Design review of the part built by this model. Coordinates are the model's own, in mm. A direction names the side the tool comes from. Coordinates: 2 decimals unless noted, no trailing zeros. Loops run counter-clockwise (first coordinate to the right, second up) from the corner with the lowest first, then second, coordinate; pieces in that order, holes last. Notation, with made-up numbers: (60.5, 6.5) - (101.5, 6.5) arc R31 cw to (101.5, 43.5) - close; hole circle Ø1 at (30.25, -35). An arc over 180 degrees is marked (long way). Return JSON: item names as keys, results as strings. Group by question number.
from build123d import *

# Parameters (mm, degrees)
BOSS_EXTRUDE1_DEPTH  = 15
SKETCH2_R            = 12.5
BOSS_EXTRUDE2_DEPTH  = 35
FILLET1_R            = 2
SKETCH3_R            = 10
BOSS_EXTRUDE3_DEPTH  = 15
FILLET1_OF_MIRROR1_R = 2


with BuildPart() as part:
    # Sketch1 → Boss-Extrude1 (new body)
    with BuildSketch(Plane.XY):
        with BuildLine():
            Line((-12.5, 50), (-12.5, 21.650635095))
            ThreePointArc((-12.5, 21.650635095), (0, -25), (12.5, 21.650635095))
            Line((12.5, 21.650635095), (12.5, 50))
            ThreePointArc((12.5, 50), (0, 62.5), (-12.5, 50))
        make_face()
    boss_extrude1 = extrude(amount=BOSS_EXTRUDE1_DEPTH)

    # Sketch2 → Boss-Extrude2 (add)
    with BuildSketch(Plane.XY.offset(15)):
        Circle(SKETCH2_R)
    boss_extrude2 = extrude(amount=BOSS_EXTRUDE2_DEPTH)

    # Fillet1
    fillet1_edges = [part.edges().sort_by_distance(p)[0] for p in [
        (-12.5, 0, 15),
    ]]
    fillet(fillet1_edges, radius=FILLET1_R)

    # Sketch3 → Boss-Extrude3 (add)
    with BuildSketch(Plane(origin=(0, 0, 0), x_dir=(-1, 0, 0), z_dir=(0, 0, -1))):
        with Locations((0, 50)):
            Circle(SKETCH3_R)
    extrude(amount=BOSS_EXTRUDE3_DEPTH)

    # Mirror1: Boss-Extrude1, Boss-Extrude2 across plane
    add(boss_extrude1.mirror(Plane.XY.offset(-7.5)))
    add(boss_extrude2.mirror(Plane.XY.offset(-7.5)))

    # Fillet1 of Mirror1
    fillet1_of_mirror1_edges = [part.edges().sort_by_distance(p)[0] for p in [
        (-12.5, 0, -30),
    ]]
    fillet(fillet1_of_mirror1_edges, radius=FILLET1_OF_MIRROR1_R)


solid = part.part
Item 1: Draft analysis for pull direction Z (two halves, no side actions). For faces 1 (the face through (0, 0, -65)), 2 (the face through (11.923, 3.755, -48.269)), 3 (the face through (0, 10, -15)), state which applies: pulls with the +Z half, pulls with the -Z half, needs draft (parallel to the pull), parting line crosses it, or undercut.
Item 2: For P1, Ø8, axis at y = 4, z = 28, coming from the +X side; P2, Ø8, axis at y = 19.5, z = 13.5, coming from the -X side; P3, Ø4.5, axis at y = 40.5, z = -21, coming from the -X side, all flat-tipped, find the tip position at first contact; note any pin that passes through.
Item 3: Add section C-C (x = 0). State the section outline as (y, z) points, then the cut area to 3 significant figures.
Item 4: Add section B-B (x = -20). State the section outline as (y, z) points, then the cut area to 3 significant figures.
Item 5: To check wall thickness, follow line 1 (Z direction, x = 10.5, y = 31); line 2 (Z direction, x = -2, y = 8); line 3 (X direction, y = 50, z = -28). State the ranges of each line that lie inside material, in increasing order. Write a range as from..to.
Item 6: For faces 4 (the face through (12.5, 36, 7)), 5 (the face through (11.923, 3.755, 33.269)), 6 (the face through (0, 19, -30)), 7 (the face through (-12.5, 36, -22)), 8 (the face through (2.17, 40.24, -7.4)), list the 3-axis set-ups (+Z, -Z, +X, -X, +Y, -Y) from which the entire face can be reached by the end or side of a thin tool; tool diameter is ignored.
Item 7: Add section D-D (y = 53.5). State the section outline as (x, z) points.
Item 8: Add section A-A (y = 0). State the section outline as (x, z) points, then the cut area to 3 significant figures.
Answers below:
{
 "1": {"face 1": "pulls with the -Z half", "face 2": "needs draft", "face 3": "undercut"},
 "2": {"P1": "stops at x = 12.5", "P2": "stops at x = -19.62", "P3": "stops at x = -12.5"},
 "3": {"outline": "(-25, -30) - (-14.5, -30) arc R2 cw to (-12.5, -32) - (-12.5, -65) - (12.5, -65) - (12.5, -32) arc R2 cw to (14.5, -30) - (62.5, -30) - (62.5, -15) - (60, -15) - (60, 0) - (62.5, 0) - (62.5, 15) - (14.5, 15) arc R2 cw to (12.5, 17) - (12.5, 50) - (-12.5, 50) - (-12.5, 17) arc R2 cw to (-14.5, 15) - (-25, 15) - (-25, 0) - (40, 0) - (40, -15) - (-25, -15) - close", "area": "4,680 mm^2"},
 "4": {"outline": "(-15, -30) - (15, -30) - (15, -15) - (-15, -15) - close; (-15, 0) - (15, 0) - (15, 15) - (-15, 15) - close", "area": "900 mm^2"},
 "5": {"line 1": "z = -30..-15, 0..15", "line 2": "z = -65..-15, 0..50", "line 3": "x = -12.5..12.5"},
 "6": {"face 4": "+Z, -Z, +X, +Y", "face 5": "+Z", "face 6": "-Z", "face 7": "+Z, -Z, -X, +Y", "face 8": "none"},
 "7": {"outline": "(-12, -30) - (12, -30) - (12, -15) - (9.37, -15) - (9.37, 0) - (12, 0) - (12, 15) - (-12, 15) - (-12, 0) - (-9.37, 0) - (-9.37, -15) - (-12, -15) - close"},
 "8": {"outline": "(-25, -30) - (-14.5, -30) arc R2 cw to (-12.5, -32) - (-12.5, -65) - (12.5, -65) - (12.5, -32) arc R2 cw to (14.5, -30) - (25, -30) - (25, -15) - (-25, -15) - close; (-25, 0) - (25, 0) - (25, 15) - (14.5, 15) arc R2 cw to (12.5, 17) - (12.5, 50) - (-12.5, 50) - (-12.5, 17) arc R2 cw to (-14.5, 15) - (-25, 15) - close", "area": "3,250 mm^2"}
}
